The listing builds one solid part. Answer for the finished solid, in the listing's coordinates (mm). Face numbers are marked on the shaded views. A direction names the side the tool comes from. Give positions to 0.01 mm unless a question says otherwise; leave off trailing zeros. Order: outer loops, then holes, each group sorted by start corner. A loop starts at its lowest first (then second) coordinate and runs counter-clockwise, first axis right, second up. Notation, with made-up numbers: (-26, 26) - (2, 26) arc R24 ccw to (2, 56) - close; hole circle Ø11 at (-25, 64.5). An arc over 180 degrees is marked (long way). Use CSV: the item, a comma, the result in double quotes.
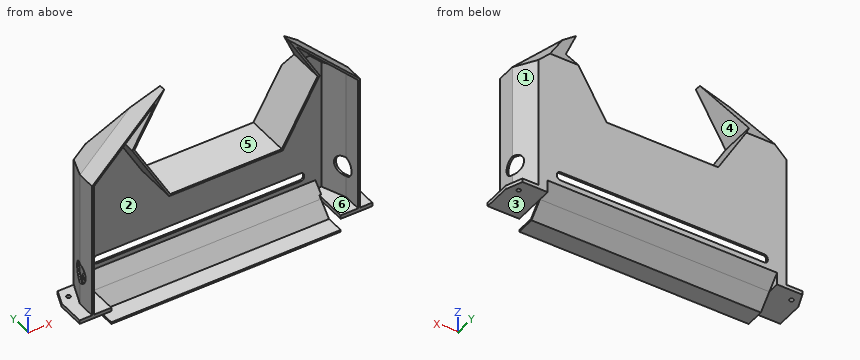
```python
from build123d import *
from OCP.BRepFilletAPI import BRepFilletAPI_MakeChamfer

# Parameters (mm, degrees)
BOSS_EXTRU_1_DEPTH           = 35
ENL_V_MAT_EXTRU_1_DEPTH      = 146.832988115
ENL_V_MAT_EXTRU_1_DEPTH_BACK = 146.832988115
CHANFREIN2_SIZE              = 20
CHANFREIN2_SIZE2             = 8.080524517
BOSS_EXTRU_2_DEPTH           = 92.5
ENL_V_MAT_EXTRU_2_DEPTH      = 185
COQUE1_T                     = -1.5
ESQUISSE5_R                  = 8
ENL_V_MAT_EXTRU_3_DEPTH      = 238.190346394
ESQUISSE6_W                  = 170
ESQUISSE6_H                  = 7
ENL_V_MAT_EXTRU_4_DEPTH      = 146.832988115
CONG_1_R                     = 3
ESQUISSE7_R                  = 1.65
BOSS_EXTRU_3_DEPTH           = 3
ENL_V_MAT_EXTRU_5_DEPTH      = 185


with BuildPart() as part:
    # Esquisse1 → Boss.-Extru.1 (new body)
    with BuildSketch(Plane(origin=(0, 0, 0), x_dir=(1, 0, 0), z_dir=(0, 1, 0))):
        Polygon((-108, -33.421356237), (-49.888518291, -91.532837946), (-73.867513459, -50), (-45, 0), (0, 0), (0, 80), (-108, 80), align=None)
    extrude(amount=BOSS_EXTRU_1_DEPTH)

    # Esquisse2 → Enlèv. mat.-Extru.1 (cut, two sides: drawn at the far end of the back side and taken through both)
    with BuildSketch(Plane(origin=(0, 0, 0), x_dir=(0, 0, -1), z_dir=(1, 0, 0)).offset(-ENL_V_MAT_EXTRU_1_DEPTH_BACK)):
        Polygon((-91.532837946, 35), (-91.532837946, 4.888518291), (-39.378221735, 35), align=None)
    extrude(amount=ENL_V_MAT_EXTRU_1_DEPTH + ENL_V_MAT_EXTRU_1_DEPTH_BACK, mode=Mode.SUBTRACT)

    # Chanfrein2: one chamfer whose edges measure the first distance from different faces: ONE call of the kernel's chamfer builder (chamfer() names one face for all edges)
    chanfrein2_edges_1 = [part.edges().sort_by_distance(p)[0] for p in [
        (-108, 35, -23.289321881),
    ]]
    chanfrein2_side_1 = [part.faces().sort_by_distance(p)[0] for p in [
        (-108, 17.5, -23.289321881),
    ]]
    chanfrein2_edges_2 = [part.edges().sort_by_distance(p)[0] for p in [
        (-105.021567251, 35, 36.399788986),
    ]]
    chanfrein2_side_2 = [part.faces().sort_by_distance(p)[0] for p in [
        (-86.283455205, 12.807012464, 55.137901032),
    ]]
    chanfrein2 = BRepFilletAPI_MakeChamfer(part.part.solid().wrapped)
    for e in chanfrein2_edges_1:
        chanfrein2.Add(CHANFREIN2_SIZE, CHANFREIN2_SIZE2, e.wrapped, chanfrein2_side_1[0].wrapped)  # the first distance lies on this face
    for e in chanfrein2_edges_2:
        chanfrein2.Add(CHANFREIN2_SIZE, CHANFREIN2_SIZE2, e.wrapped, chanfrein2_side_2[0].wrapped)  # the first distance lies on this face
    add(Compound.cast(chanfrein2.Shape()), mode=Mode.REPLACE)

    # Symétrie1: part across plane


with BuildPart() as part_1:
    add(part.part)
    add(part.part.mirror(Plane(origin=(0, 35, -80), x_dir=(0, 0, 1), z_dir=(-1, 0, 0))))

    # Esquisse3 → Boss.-Extru.2 (add, symmetric)
    with BuildSketch(Plane(origin=(0, 0, 0), x_dir=(0, 0, -1), z_dir=(1, 0, 0))):
        Polygon((80, 25.476190476), (91, 15), (91, 0), (80, 0), align=None)
    extrude(amount=BOSS_EXTRU_2_DEPTH, both=True)

    # Esquisse4 → Enlèv. mat.-Extru.2 (cut)
    with BuildSketch(Plane(origin=(92.5, 0, 0), x_dir=(0, 0, -1), z_dir=(1, 0, 0))):
        Polygon((91, 15), (70, 35), (91, 35), align=None)
    extrude(amount=-ENL_V_MAT_EXTRU_2_DEPTH, mode=Mode.SUBTRACT)

    # Coque1
    coque1_openings = [part_1.faces().sort_by_distance(p)[0] for p in [
        (0, 0, -29.297783108),
    ]]
    offset(amount=COQUE1_T, openings=coque1_openings, kind=Kind.INTERSECTION)

    # Esquisse5 → Enlèv. mat.-Extru.3 (cut, through all)
    with BuildSketch(Plane.ZY.offset(108)):
        with Locations(Location((-51, 16, 0), (0, 0, 352.819244219))):
            Circle(ESQUISSE5_R)
    extrude(amount=-ENL_V_MAT_EXTRU_3_DEPTH, mode=Mode.SUBTRACT)

    # Esquisse6 → Enlèv. mat.-Extru.4 (cut, through all)
    with BuildSketch(Plane(origin=(0, 35, 0), x_dir=(1, 0, 0), z_dir=(0, 1, 0))):
        with Locations((0, 62)):
            Rectangle(ESQUISSE6_W, ESQUISSE6_H)
    extrude(amount=-ENL_V_MAT_EXTRU_4_DEPTH, mode=Mode.SUBTRACT)

    # Congé1
    cong_1_edges = [part_1.edges().sort_by_distance(p)[0] for p in [
        (85, 34.25, -65.5),
        (85, 34.25, -58.5),
        (-85, 34.25, -58.5),
        (-85, 34.25, -65.5),
    ]]
    fillet(cong_1_edges, radius=CONG_1_R)

    # Esquisse7 → Boss.-Extru.3 (add)
    # profile 1 of 2: a face of its own
    with BuildSketch(Plane(origin=(0, 0, -80), x_dir=(-1, 0, 0), z_dir=(0, 0, -1))):
        Polygon((-92.5, 0), (-118, 0), (-118, 22.282737416), (-112.861892395, 35), (-92.5, 35), align=None)
        with Locations((-110, 26.066629268)):
            Circle(ESQUISSE7_R, mode=Mode.SUBTRACT)
    # profile 2 of 2: a face of its own
    with BuildSketch(Plane(origin=(0, 0, -80), x_dir=(-1, 0, 0), z_dir=(0, 0, -1))):
        Polygon((92.5, 0), (118, 0), (118, 22.282737416), (112.861892395, 35), (92.5, 35), align=None)
        with Locations(Location((110, 26.066629268, 0), (0, 0, 180))):
            Circle(ESQUISSE7_R, mode=Mode.SUBTRACT)
    extrude(amount=-BOSS_EXTRU_3_DEPTH)

    # Esquisse8 → Enlèv. mat.-Extru.5 (cut)
    with BuildSketch(Plane.ZY.offset(-92.5)):
        Polygon((-78.5, 0), (-78.5, 24.833333333), (-89.5, 14.357142857), (-89.5, 0), align=None)
    extrude(amount=ENL_V_MAT_EXTRU_5_DEPTH, mode=Mode.SUBTRACT)


solid = part_1.part
```
Item 1: The part is cut by section C-C (z = 10). Give the vertices of the cut face in (x, y), and give its area (3 significant figures).
Taken from the geometry:
outline,"(-108, 0) - (-106.5, 0) - (-106.5, 14.71) - (-98.91, 33.5) - (-52.51, 33.5) - (-52.51, 0) - (-50.77, 0) - (-50.77, 35) - (-99.92, 35) - (-108, 15) - close; (50.77, 0) - (52.51, 0) - (52.51, 33.5) - (98.91, 33.5) - (106.5, 14.71) - (106.5, 0) - (108, 0) - (108, 15) - (99.92, 35) - (50.77, 35) - close"
area,"369 mm^2"
Item 2: The part is cut by section A-A (x = -3.5). Give the vertices of the cut face in (y, z), and give its area (3 significant figures).
Taken from the geometry:
outline,"(0, -91) - (15, -91) - (35, -70) - (35, -65.5) - (33.5, -65.5) - (33.5, -69.4) - (14.36, -89.5) - (0, -89.5) - close; (0, -1.5) - (33.5, -1.5) - (33.5, -58.5) - (35, -58.5) - (35, 0) - (0, 0) - close"
area,"209 mm^2"
Item 3: The part is cut by section B-B (z = -51). Give the vertices of the cut face in (x, y), and give its area (3 significant figures).
Taken from the geometry:
outline,"(-108, 0) - (-106.5, 0) - (-106.5, 8) - (-108, 8) - close; (-104.36, 24) - (-102.75, 24) - (-98.91, 33.5) - (98.91, 33.5) - (102.75, 24) - (104.36, 24) - (99.92, 35) - (-99.92, 35) - close; (106.5, 0) - (108, 0) - (108, 8) - (106.5, 8) - close"
area,"355 mm^2"
Item 4: Each of these flat-tipped pins is pushed along its axis until it touches: pin 1 (8 mm diameter, centred on y = 15.5, z = -4, fed in from +X); pin 2 (3 mm diameter, centred on y = 25, z = 19.5, fed in from +X); pin 3 (1.5 mm diameter, centred on y = 8, z = -6, fed in from -X). Where does it stop, or does it pass through?
Taken from the geometry:
pin 1,"x = 108"
pin 2,"x = 104.57"
pin 3,"x = -108"
Item 5: Find the intervals of material crossed by line 1 along X through (y, z) = (4, -18); line 2 along Y through (x, z) = (-110, -78); line 3 along X through (y, z) = (19, 21.5), in increasing order.
Taken from the geometry:
line 1,"-108 to -106.5, 106.5 to 108"
line 2,"0 to 24.42, 27.72 to 35"
line 3,"-106.38 to -104.77, -59.15 to -57.41, 57.41 to 59.15, 104.77 to 106.38"
Item 6: The part is cut by section D-D (z = -21.5). Give the vertices of the cut face in (x, y).
Taken from the geometry:
outline,"(-108, 0) - (-106.5, 0) - (-106.5, 14.71) - (-98.91, 33.5) - (98.91, 33.5) - (106.5, 14.71) - (106.5, 0) - (108, 0) - (108, 15) - (99.92, 35) - (-99.92, 35) - (-108, 15) - close"
Item 7: Which of the six approach directions +Z, -Z, +X, -X, +Y, -Y give full straight-line access (tool end or side, diameter ignored) to the marked faces 4, 5 and 6?
Taken from the geometry:
face 4,"+Y, -Y"
face 5,"+Z, +Y, -Y"
face 6,"-Y"
Item 8: The mould has two halves that part along X. Classify the marked faces 1, 2 and 3: +X half, -X half, draft (parallel to the pull), parting line (faces both ways), or undercut.
Taken from the geometry:
face 1,"+X half"
face 2,"undercut"
face 3,"draft"
